```python
from build123d import *

# Parameters (mm, degrees)
BOSS_EXTRUDE1_DEPTH = 17.5
CHAMFER1_SIZE       = 3
BOSS_EXTRUDE2_DEPTH = 5
CHAMFER2_SIZE       = 8
SKETCH3_R           = 1.5
CUT_EXTRUDE1_DEPTH  = 33.035136959
FILLET1_R           = 3
SKETCH4_R           = 1
CUT_EXTRUDE2_DEPTH  = 8
BOSS_EXTRUDE3_DEPTH = 12.5


with BuildPart() as part:
    # Sketch1 → Boss-Extrude1 (new body)
    with BuildSketch(Plane.XY):
        Polygon((12, -12), (16, -12), (16, 4), (-16, 4), (-16, -12), (-12, -12), (-12, 0), (12, 0), align=None)
    extrude(amount=BOSS_EXTRUDE1_DEPTH)

    # Chamfer1
    chamfer1_edges = [part.edges().sort_by_distance(p)[0] for p in [
        (-16, 4, 8.75),
        (16, 4, 8.75),
    ]]
    chamfer(chamfer1_edges, length=CHAMFER1_SIZE)

    # Sketch2 → Boss-Extrude2 (add)
    with BuildSketch(Plane.XY.offset(17.5)):
        Polygon((-16, 1), (-4, 1), (-4, 9), (-16, 9), (-24, 9), (-24, -12), (-16, -12), align=None)
    extrude(amount=-BOSS_EXTRUDE2_DEPTH)

    # Chamfer2
    chamfer2_edges = [part.edges().sort_by_distance(p)[0] for p in [
        (-24, -12, 15),
    ]]
    chamfer(chamfer2_edges, length=CHAMFER2_SIZE)

    # Sketch3 → Cut-Extrude1 (cut, through all)
    with BuildSketch(Plane.XY.offset(17.5)):
        with Locations((-21, 6)):
            Circle(SKETCH3_R)
    extrude(amount=-CUT_EXTRUDE1_DEPTH, mode=Mode.SUBTRACT)

    # Fillet1
    fillet1_edges = [part.edges().sort_by_distance(p)[0] for p in [
        (-24, 9, 15),
    ]]
    fillet(fillet1_edges, radius=FILLET1_R)

    # Sketch4 → Cut-Extrude2 (cut)
    with BuildSketch(Plane(origin=(0, 0, 0), x_dir=(-1, 0, 0), z_dir=(0, 0, -1))):
        with Locations((-14.5, -6)):
            Circle(SKETCH4_R)
        with Locations((14.5, -6)):
            Circle(SKETCH4_R)
    extrude(amount=-CUT_EXTRUDE2_DEPTH, mode=Mode.SUBTRACT)

    # Sketch5 → Boss-Extrude3 (add)
    with BuildSketch(Plane(origin=(0, 0, 0), x_dir=(-1, 0, 0), z_dir=(0, 0, -1))):
        with BuildLine():
            Line((13, 4), (16, 1))
            Line((16, 1), (16, -12))
            Line((16, -12), (24, -4))
            Line((24, -4), (24, -2))
            ThreePointArc((24, -2), (19.264982043, 2.402467079), (13, 4))
        make_face()
    extrude(amount=-BOSS_EXTRUDE3_DEPTH)


solid = part.part
```
Geometry check sheet. Reference: the model listing, model coordinates, mm. A direction names the side the tool comes from. Coordinates: 2 decimals unless noted, no trailing zeros. Loops run counter-clockwise (first coordinate to the right, second up) from the corner with the lowest first, then second, coordinate; pieces in that order, holes last.
Item 1: Go/stop test with flat-tipped pins: pin 1 Ø4 at (y, z) = (6.5, 14) entering from +X; pin 2 Ø3.5 at (y, z) = (-8, 11) entering from -X; pin 3 Ø9 at (x, z) = (-2.5, 7.5) entering from -Y. Record where each tip stops, or that it passes through.
Item 2: Thickness scan on line 1 (Y direction, x = -21, z = 14); line 2 (Y direction, x = 8.5, z = 10.5); line 3 (Z direction, x = -8.5, y = 7.5). Record the ranges inside material, lowest first.
Item 3: Access from +Z, -Z, +X, -X, +Y, -Y to the whole of each face (thin tool, end or side, straight path). Record for faces 1 (the face through (-4, 6, 15)), 2 (the face through (-19.345, 2.358, 6.162)), 3 (the face through (-15.454, -5.7, 3.944)).
Item 4: Sectioned sample at C-C, the plane y = -8. Record the boundary of the cut face in (x, z), then the cut area to 3 significant figures.
Item 5: Sectioned sample at B-B, the plane x = 14.5. Record the boundary of the cut face in (y, z), then the cut area to 3 significant figures.
Item 6: Sectioned sample at A-A, the plane z = 2. Record the boundary of the cut face in (x, y).
Item 7: Release check for a two-part mould opening along Y. For faces 4 (the face through (-12, 9, 15)), 5 (the face through (13.546, -5.7, 3.944)), 6 (the face through (15, -6, 8)), 7 (the face through (0, 0, 9)) record: released by +Y, released by -Y, zero draft, split by the parting line, or undercut.
Item 8: Sectioned sample at D-D, the plane z = 13. Record the boundary of the cut face in (x, y), then the cut area to 4 significant figures.
Check result:
1. pin 1: stops at x = -4
1. pin 2: stops at x = -21.75
1. pin 3: stops at y = 0
2. line 1: y = -7 to 4.5, 7.5 to 9
2. line 2: y = 0 to 4
2. line 3: z = 12.5 to 17.5
3. face 1: +Z, -Z, +X, +Y
3. face 2: -Z, -X, +Y
3. face 3: -Z
4. outline: (-20, 0) - (-12, 0) - (-12, 17.5) - (-20, 17.5) - close; (12, 0) - (16, 0) - (16, 17.5) - (12, 17.5) - close
4. area: 210 mm2
5. outline: (-12, 0) - (-7, 0) - (-7, 8) - (-5, 8) - (-5, 0) - (2.5, 0) - (2.5, 17.5) - (-12, 17.5) - close
5. area: 238 mm2
6. outline: (-24, -4) - (-16, -12) - (-12, -12) - (-12, 0) - (12, 0) - (12, -12) - (16, -12) - (16, 1) - (13, 4) - (-13, 4) arc R13.08 ccw to (-24, -2) - close; hole circle Ø2 at (-14.5, -6); hole circle Ø2 at (14.5, -6)
7. face 4: released by +Y
7. face 5: undercut
7. face 6: undercut
7. face 7: released by -Y
8. outline: (-24, -4) - (-16, -12) - (-12, -12) - (-12, 0) - (12, 0) - (12, -12) - (16, -12) - (16, 1) - (13, 4) - (-4, 4) - (-4, 9) - (-21, 9) arc R3 ccw to (-24, 6) - close; hole circle Ø3 at (-21, 6)
8. area: 406.5 mm2
